from build123d import *

# Parameters (mm, degrees)
SKETCH1_W            = 76.2
SKETCH1_H            = 16.378
BOSS_EXTRUDE1_DEPTH  = 3.175
FILLET1_R            = 2
M8_CLEARANCE_HOLE1_D = 9


with BuildPart() as part:
    # Sketch1 → Boss-Extrude1 (new body)
    with BuildSketch(Plane.XY):
        with Locations((38.1, -8.189)):
            Rectangle(SKETCH1_W, SKETCH1_H)
    extrude(amount=BOSS_EXTRUDE1_DEPTH)

    # Fillet1
    fillet1_edges = [part.edges().sort_by_distance(p)[0] for p in [
        (0, 0, 1.5875),
        (76.2, 0, 1.5875),
        (76.2, -16.378, 1.5875),
        (0, -16.378, 1.5875),
    ]]
    fillet(fillet1_edges, radius=FILLET1_R)

    # M8 Clearance Hole1 (through all)
    with Locations(Plane.XY.offset(3.175)):
        with Locations((10, -8.189)):
            Hole(M8_CLEARANCE_HOLE1_D / 2)


solid = part.part
Verification items for the finished model (mm, model axes). Coordinates: 2 decimals unless noted, no trailing zeros. Write each loop counter-clockwise with the first axis right and the second up, starting at its lowest first coordinate (ties: lowest second). Pieces come first, ordered by that corner, then holes. Notation, with made-up numbers: M 81,-5.75 L 129,-5.75 A20 ccw 129,-1.75 Z; hole C 59,-7 d8. An arc over 180 degrees is marked long. Use a Markdown table: item, result.
Q1. Sectioned sample at A-A, the plane x = 10. Record the boundary of the cut face in (y, z) (3 decimals).
Reply:
| item | result |
|---|---|
| outline | M -16.378,0 L -12.689,0 L -12.689,3.175 L -16.378,3.175 Z; M -3.689,0 L 0,0 L 0,3.175 L -3.689,3.175 Z |
Q2. Sectioned sample at B-B, the plane y = -5. Record the boundary of the cut face in (x, z) (3 decimals), plus the area to 3 significant figures.
Reply:
| item | result |
|---|---|
| outline | M 0,0 L 6.825,0 L 6.825,3.175 L 0,3.175 Z; M 13.175,0 L 76.2,0 L 76.2,3.175 L 13.175,3.175 Z |
| area | 222 mm² |
Q3. Sectioned sample at C-C, the plane z = 2.35. Record the boundary of the cut face in (x, y).
Reply:
| item | result |
|---|---|
| outline | M 0,-14.38 A2 ccw 2,-16.38 L 74.2,-16.38 A2 ccw 76.2,-14.38 L 76.2,-2 A2 ccw 74.2,0 L 2,0 A2 ccw 0,-2 Z; hole C 10,-8.19 d9 |
Q4. Draft check along Y on faces 1 (the face through (5.708, -6.837, 1.565)), 2 (the face through (38, -8, 3.175)), 3 (the face through (38, -16.378, 2)). Enter one of: +Y half, -Y half, draft (parallel to the pull), parting line (faces both ways), or undercut.
Reply:
| item | result |
|---|---|
| face 1 | undercut |
| face 2 | draft |
| face 3 | -Y half |
Q5. Thickness scan on line 1 (Y direction, x = 10, z = 1.45); line 2 (X direction, y = -6.25, z = 1); line 3 (X direction, y = -10.5, z = 0.5). Record the ranges inside material, lowest first.
Reply:
| item | result |
|---|---|
| line 1 | y = -16.38 to -12.69, -3.69 to 0 |
| line 2 | x = 0 to 5.94, 14.06 to 76.2 |
| line 3 | x = 0 to 6.14, 13.86 to 76.2 |
